Geometry check sheet. Reference: the model listing, model coordinates, mm. A direction names the side the tool comes from. Coordinates: 2 decimals unless noted, no trailing zeros. Loops run counter-clockwise (first coordinate to the right, second up) from the corner with the lowest first, then second, coordinate; pieces in that order, holes last. Notation, with made-up numbers: (18.25, -18.5) - (60.25, -18.5) arc R31 cw to (60.25, 13.5) - close; hole circle Ø11 at (75, 73). An arc over 180 degrees is marked (long way). Write item = value, one per line. Start each with the question number.
Autodesk Inventor part; units mm, degrees
ref_plane "YZ Plane" through (0, 0, 0) normal (1, 0, 0) x (0, 1, 0)
ref_plane "XZ Plane" through (0, 0, 0) normal (0, 1, 0) x (-1, 0, 0)
ref_plane "XY Plane" through (0, 0, 0) normal (0, 0, 1) x (1, 0, 0)
sketch "Sketch1" plane through (0, 0, 0) normal (0, 0, 1) x (1, 0, 0)
  line L0 (-6.8, -3.1) -> (-5.8439, -3.1)
  arc A0 (-5.8439, -5.5) -> (-5.8439, -3.1) centre (-4, -4.3) ccw
  line L1 (-5.8439, -5.5) -> (-6.8, -5.5)
  line L2 (-6.8, -5.5) -> (-6.8, -3.1)
  line L3 (-6.8, -16.9) -> (-6.8, -14.5)
  line L4 (-5.8439, -14.5) -> (-6.8, -14.5)
  arc A1 (-5.8439, -16.9) -> (-5.8439, -14.5) centre (-4, -15.7) ccw
  line L5 (-5.8439, -16.9) -> (-6.8, -16.9)
  arc A2 (47.1, 2) -> (44.1, 5) centre (44.1, 2) ccw
  line L6 (44.1, 5) -> (-5.8, 5)
  arc A3 (-5.8, 5) -> (-8.8, 2) centre (-5.8, 2) ccw
  line L7 (-8.8, -3.3038) -> (-8.8, 2)
  spline S0 degree 3 poles (-11.8, -8.5) (-11.3844, -8.0844) (-10.926, -7.6277) (-10.0868, -6.6554) (-9.7097, -6.1367) (-9.2499, -5.2825) (-9.0837, -4.8972) (-8.8584, -4.0991) (-8.8, -3.6862) (-8.8, -3.3038) knots 0 0 0 0 0.176344 0.176344 0.352688 0.352688 0.467383 0.467383 0.582078 0.582078 0.582078 0.582078
  line L8 (-71, -8.5) -> (-11.8, -8.5)
  arc A4 (-71, -11.5) -> (-71, -8.5) centre (-71.8, -10) ccw
  line L9 (-11.8, -11.5) -> (-71, -11.5)
  spline S1 degree 3 poles (-8.8, -16.6962) (-8.8, -16.3138) (-8.8584, -15.9009) (-9.0837, -15.1028) (-9.2499, -14.7175) (-9.7097, -13.8633) (-10.0868, -13.3446) (-10.926, -12.3723) (-11.3844, -11.9156) (-11.8, -11.5) knots 1.516597 1.516597 1.516597 1.516597 1.631292 1.631292 1.745986 1.745986 1.922331 1.922331 2.098675 2.098675 2.098675 2.098675
  line L10 (-8.8, -17) -> (-8.8, -16.6962)
  arc A5 (-8.8, -17) -> (-5.8, -20) centre (-5.8, -17) ccw
  line L11 (-5.8, -20) -> (0, -20)
  line L12 (0, -20) -> (0, 0)
  line L13 (0, 0) -> (40.3, 0)
  line L14 (40.3, -20) -> (40.3, 0)
  line L15 (47.1, -20) -> (40.3, -20)
  line L16 (47.1, -16.9) -> (47.1, -20)
  line L17 (47.1, -16.9) -> (46.1439, -16.9)
  arc A6 (46.1439, -14.5) -> (46.1439, -16.9) centre (44.3, -15.7) ccw
  line L18 (46.1439, -14.5) -> (47.1, -14.5)
  line L19 (47.1, -5.5) -> (47.1, -14.5)
  line L20 (47.1, -5.5) -> (46.1439, -5.5)
  arc A7 (46.1439, -3.1) -> (46.1439, -5.5) centre (44.3, -4.3) ccw
  line L21 (46.1439, -3.1) -> (47.1, -3.1)
  line L22 (47.1, -3.1) -> (47.1, 2)
extrude "Extrusion1" add sketch "Sketch1" along normal blind 1
sketch "Sketch2" plane through (0, 0, 1) normal (0, 0, 1) x (1, 0, 0)
  line L0 (-6.8, -14.5) -> (-5.8439, -14.5)
  arc A0 (-5.8439, -16.9) -> (-5.8439, -14.5) centre (-4, -15.7) ccw
  line L1 (-5.8439, -16.9) -> (-6.8, -16.9)
  line L2 (-6.8, -16.9) -> (-6.8, -14.5)
  arc A1 (-5.8439, -5.5) -> (-5.8439, -3.1) centre (-4, -4.3) ccw
  line L3 (-5.8439, -5.5) -> (-6.8, -5.5)
  line L4 (-6.8, -5.5) -> (-6.8, -3.1)
  line L5 (-6.8, -3.1) -> (-5.8439, -3.1)
  line L6 (-1.8, 10.0452) -> (-75.924, 10.0452)
  line L7 (-75.924, 10.0452) -> (-75.924, -24.7516)
  line L8 (-75.924, -24.7516) -> (-1.8, -24.7516)
  line L9 (-1.8, -24.7516) -> (-1.8, 10.0452)
  line L10 (42.1, 14.1949) -> (61.4451, 14.1949)
  line L11 (61.4451, 14.1949) -> (61.4451, -26.9512)
  line L12 (61.4451, -26.9512) -> (42.1, -26.9512)
  line L13 (42.1, -26.9512) -> (42.1, 14.1949)
extrude "Extrusion2" cut sketch "Sketch2" against normal blind 1
sketch "Sketch3" plane through (0, -20, 0) normal (1, 0, 0) x (0, 0, -1)
  line L0 (0, 0) -> (0, 20)
  line L1 (0, 20) -> (-1, 20)
  line L2 (-1, 0) -> (-1, 20)
  line L3 (0, 0) -> (-1, 0)
extrude "Extrusion3" cut sketch "Sketch3" against normal blind 0.25
sketch "Sketch4" plane through (40.3, -20, 0) normal (-1, 0, 0) x (0, 0, 1)
  line L0 (0, 20) -> (0, 0)
  line L1 (0, 0) -> (1, 0)
  line L2 (1, 20) -> (1, 0)
  line L3 (0, 20) -> (1, 20)
extrude "Extrusion4" cut sketch "Sketch4" against normal blind 0.25
properties part number "Fork2DimTest"
(1) Sectioned sample at A-A on y = -16. Enter the section's corners in (x, z), plus the area to 3 significant figures.
(2) Scan lines: line 1 (X direction, y = -18, z = 0.1); line 2 (Y direction, x = 4, z = 0.8). Record each from-to range of solid material in increasing order.
(3) Tool access check on faces 1 (the face through (19.9, 0, 0.5)), 2 (the face through (20.5, 5, 0.5)). Record the directions out of +Z, -Z, +X, -X, +Y, -Y that give a thin tool (end or side, any length) a straight path to the whole face; none if there is none.
(4) Depth check by flat-ended pin: pin 1 (0.5 mm diameter, centred on x = 16.5, z = 0.5, fed in from -Y). Enter the tip coordinate at first touch or a pass-through.
(5) Draft check along X on faces 3 (the face through (41.3, -20, 0.5)), 4 (the face through (40.55, -9.9, 0.5)), 5 (the face through (42.1, -7.7, 0.5)). Enter one of: pulls with the +X half, pulls with the -X half, needs draft (parallel to the pull), parting line crosses it, or undercut.
(6) Sectioned sample at B-B on z = 0.25. Enter the section's corners in (x, y), plus the area to 4 significant figures.
(7) Sectioned sample at C-C on x = 3.5. Enter the section's corners in (y, z), plus the area to 3 significant figures.
Working result:
q1.outline = (-1.8, 0) - (-0.25, 0) - (-0.25, 1) - (-1.8, 1) - close; (40.55, 0) - (42.1, 0) - (42.1, 1) - (40.55, 1) - close
q1.area = 3.10 mm2
q2.line_1 = -1.8 to -0.25, 40.55 to 42.1
q2.line_2 = 0 to 5
q3.face_1 = +Z, -Z, -Y
q3.face_2 = +Z, -Z, +X, -X, +Y
q4.pin_1 = 0
q5.face_3 = needs draft
q5.face_4 = undercut
q5.face_5 = pulls with the +X half
q6.outline = (-1.8, -20) - (-0.25, -20) - (-0.25, 0) - (40.55, 0) - (40.55, -20) - (42.1, -20) - (42.1, 5) - (-1.8, 5) - close
q6.area = 281.5 mm2
q7.outline = (0, 0) - (5, 0) - (5, 1) - (0, 1) - close
q7.area = 5.00 mm2
